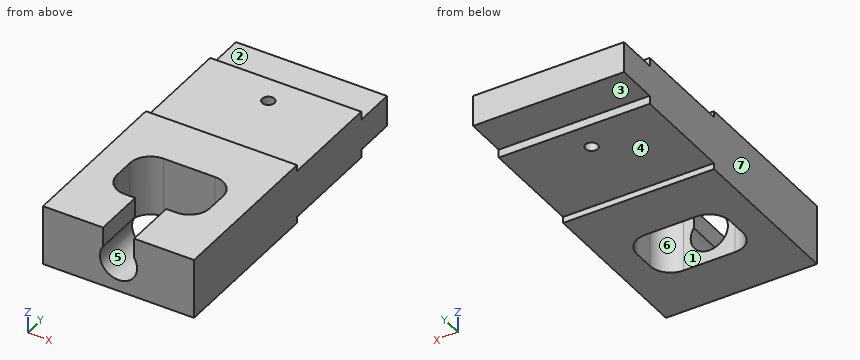
```python
from build123d import *

# Parameters (mm, degrees)
F2_DEPTH = 7.3
F3_R     = 0.3
F4_DEPTH = 2.901
F6_DEPTH = 2.5


with BuildPart() as f2:
    # F1 (on Right) → F2 (new body)
    with BuildSketch(Plane.YZ):
        Polygon((0, 1.45), (0, 0), (0, -1.45), (8, -1.45), (8, -1.15), (13, -1.15), (13, -0.75), (15, -0.75), (15, 0), (15, 0.75), (13, 0.75), (13, 1.15), (8, 1.15), (8, 1.45), align=None)
    extrude(amount=F2_DEPTH)

    # F3 (on face) → F4 (cut, through all)
    with BuildSketch(Plane.XY.offset(1.45)):
        with BuildLine():
            ThreePointArc((1.4, 3.5), (1.6928932188, 2.7928932188), (2.4, 2.5))
            Line((2.4, 2.5), (4.9, 2.5))
            ThreePointArc((4.9, 2.5), (5.6071067812, 2.7928932188), (5.9, 3.5))
            Line((5.9, 3.5), (5.9, 4.5))
            ThreePointArc((5.9, 4.5), (5.6071067812, 5.2071067812), (4.9, 5.5))
            Line((4.9, 5.5), (2.4, 5.5))
            ThreePointArc((2.4, 5.5), (1.6928932188, 5.2071067812), (1.4, 4.5))
            Line((1.4, 4.5), (1.4, 3.5))
        make_face()
        with Locations((3.65, 11.65)):
            Circle(F3_R)
    extrude(amount=-F4_DEPTH, mode=Mode.SUBTRACT)

    # F5 (on face) → F6 (cut, through all)
    with BuildSketch(Plane.XZ):
        with BuildLine():
            Line((4.4, 1.45), (2.9, 1.45))
            Line((2.9, 1.45), (2.9, 0.4974937186))
            ThreePointArc((2.9, 0.4974937186), (3.65, -0.9), (4.4, 0.4974937186))
            Line((4.4, 0.4974937186), (4.4, 1.45))
        make_face()
    extrude(amount=-F6_DEPTH, mode=Mode.SUBTRACT)


solid = f2.part
```
Can you work these out from the model? Positions are in its coordinate system, mm. Face numbers are marked on the shaded views. A direction names the side the tool comes from. Give positions to 0.01 mm unless a question says otherwise; leave off trailing zeros. Loops run counter-clockwise (first coordinate to the right, second up) from the corner with the lowest first, then second, coordinate; pieces in that order, holes last. Notation, with made-up numbers: M 84.25,-6.75 L 91.25,-6.75 A18 ccw 91.25,6.25 Z; hole C 4.25,69.25 d9. An arc over 180 degrees is marked long. Answer in a Markdown table with one row per item.
1. Suppose I cut it at B-B on z = 0. Write out the boundary of the cut face in (x, y), plus the area to 3 significant figures.
Taken from the geometry:
| item | result |
|---|---|
| outline | M 0,0 L 2.75,0 L 2.75,2.5 L 2.4,2.5 A1 cw 1.4,3.5 L 1.4,4.5 A1 cw 2.4,5.5 L 4.9,5.5 A1 cw 5.9,4.5 L 5.9,3.5 A1 cw 4.9,2.5 L 4.55,2.5 L 4.55,0 L 7.3,0 L 7.3,15 L 0,15 Z; hole C 3.65,11.65 d0.6 |
| area | 92.1 mm² |
2. Suppose I cut it at A-A on x = 3.65. Write out the boundary of the cut face in (y, z), plus the area to 3 significant figures.
Taken from the geometry:
| item | result |
|---|---|
| outline | M 0,-1.45 L 2.5,-1.45 L 2.5,-0.9 L 0,-0.9 Z; M 5.5,-1.45 L 8,-1.45 L 8,-1.15 L 11.35,-1.15 L 11.35,1.15 L 8,1.15 L 8,1.45 L 5.5,1.45 Z; M 11.95,-1.15 L 13,-1.15 L 13,-0.75 L 15,-0.75 L 15,0.75 L 13,0.75 L 13,1.15 L 11.95,1.15 Z |
| area | 21.7 mm² |
3. Suppose I cut it at D-D on x = 5.25. Write out the boundary of the cut face in (y, z), plus the area to 3 significant figures.
Taken from the geometry:
| item | result |
|---|---|
| outline | M 0,-1.45 L 2.56,-1.45 L 2.56,1.45 L 0,1.45 Z; M 5.44,-1.45 L 8,-1.45 L 8,-1.15 L 13,-1.15 L 13,-0.75 L 15,-0.75 L 15,0.75 L 13,0.75 L 13,1.15 L 8,1.15 L 8,1.45 L 5.44,1.45 Z |
| area | 29.4 mm² |
4. Thinking about a two-plate mould opening in X: for the marked faces 4, 5, 6 and 7, which applies, released by +X, released by -X, zero draft, split by the parting line, or undercut?
Taken from the geometry:
| item | result |
|---|---|
| face 4 | zero draft |
| face 5 | undercut |
| face 6 | undercut |
| face 7 | released by -X |
5. Suppose I cut it at C-C on y = 11.65. Write out the boundary of the cut face in (x, z), plus the area to 3 significant figures.
Taken from the geometry:
| item | result |
|---|---|
| outline | M 0,-1.15 L 3.35,-1.15 L 3.35,1.15 L 0,1.15 Z; M 3.95,-1.15 L 7.3,-1.15 L 7.3,1.15 L 3.95,1.15 Z |
| area | 15.4 mm² |
6. If I drill on line 1 along X through (y, z) = (1.5, 0); line 2 along Y through (x, z) = (3.65, -0.1); line 3 along X through (y, z) = (4.25, -1), over which ranges is the centre line in solid material (lowest first)?
Taken from the geometry:
| item | result |
|---|---|
| line 1 | x = 0 to 2.75, 4.55 to 7.3 |
| line 2 | y = 5.5 to 11.35, 11.95 to 15 |
| line 3 | x = 0 to 1.4, 5.9 to 7.3 |
7. For pin 1 Ø3 at (x, y) = (1.5, 4.5) entering from -Z; pin 2 Ø4 at (x, y) = (2.5, 11.5) entering from +Z; pin 3 Ø1 at (x, y) = (4.5, 14.5) entering from -Z; pin 4 Ø1 at (x, y) = (6.5, 9) entering from -Z, each with a flat end and sliding along its axis, tell me the tip position at first contact or that it passes through.
Taken from the geometry:
| item | result |
|---|---|
| pin 1 | stops at z = -1.45 |
| pin 2 | stops at z = 1.15 |
| pin 3 | stops at z = -0.75 |
| pin 4 | stops at z = -1.15 |
8. Which directions (+Z, -Z, +X, -X, +Y, -Y) give clear straight access to the entire face, cutting with the end or side of a thin tool? Please do the marked faces 1, 2 and 3.
Taken from the geometry:
| item | result |
|---|---|
| face 1 | +Z, -Z |
| face 2 | +Z, +X, -X, +Y |
| face 3 | -Z, +X, -X, +Y |
